```python
from build123d import *

# Parameters (mm, degrees)
BOSS_EXTRUDE1_DEPTH = 90
CUT_EXTRUDE1_DEPTH  = 385.317577012
SHELL3_T            = -10
BOSS_EXTRUDE2_START = -10
BOSS_EXTRUDE2_DEPTH = 10
SKETCH9_W           = 180
SKETCH9_H           = 60
BOSS_EXTRUDE3_DEPTH = 220
SKETCH9_4_W         = 180
SKETCH9_4_H         = 60
CUT_EXTRUDE3_DEPTH  = 200
SKETCH9_5_W         = 180
SKETCH9_5_H         = 60
BOSS_EXTRUDE5_DEPTH = 10
SKETCH10_W          = 190
SKETCH10_H          = 180
BOSS_EXTRUDE6_DEPTH = 70
SKETCH10_2_W        = 190
SKETCH10_2_H        = 180
CUT_EXTRUDE4_DEPTH  = 30
SKETCH10_3_W        = 190
SKETCH10_3_H        = 180
CUT_EXTRUDE5_DEPTH  = 50
SKETCH10_4_W        = 190
SKETCH10_4_H        = 180
CUT_EXTRUDE6_DEPTH  = 60


with BuildPart() as part:
    # Sketch1 → Boss-Extrude1 (new body)
    with BuildSketch(Plane(origin=(0, 0, 0), x_dir=(1, 0, 0), z_dir=(0, 1, 0))):
        with BuildLine():
            Line((0, 100), (0, -100))
            Line((0, -100), (200, -100))
            ThreePointArc((200, -100), (294.339811321, -72.943698113), (360, 0))
            ThreePointArc((360, 0), (294.339811321, 72.943698113), (200, 100))
            Line((200, 100), (0, 100))
        make_face()
    extrude(amount=BOSS_EXTRUDE1_DEPTH)

    # Sketch2 → Cut-Extrude1 (cut, through all)
    with BuildSketch(Plane.ZY):
        Polygon((-100, 0), (0, 0), (-100, 20), align=None)
        Polygon((0, 0), (100, 20), (100, 0), align=None)
    extrude(amount=-CUT_EXTRUDE1_DEPTH, mode=Mode.SUBTRACT)

    # Shell3
    shell3_openings = [part.faces().sort_by_distance(p)[0] for p in [
        (159.417640867, 90, 0),
    ]]
    offset(amount=SHELL3_T, openings=shell3_openings, kind=Kind.INTERSECTION)

    # Sketch6 → Boss-Extrude2 (add)
    with BuildSketch(Plane(origin=(0, 90, 0), x_dir=(1, 0, 0), z_dir=(0, 1, 0)).offset(BOSS_EXTRUDE2_START)):
        with BuildLine():
            Line((200, 90), (200, -90))
            ThreePointArc((200, -90), (286.948260477, -65.749782609), (348.795161212, 0))
            ThreePointArc((348.795161212, 0), (286.948260477, 65.749782609), (200, 90))
        make_face()
    extrude(amount=BOSS_EXTRUDE2_DEPTH)

    # Sketch9 → Boss-Extrude3 (add)
    with BuildSketch(Plane.ZY):
        with Locations((0, 50)):
            Rectangle(SKETCH9_W, SKETCH9_H)
    extrude(amount=-BOSS_EXTRUDE3_DEPTH)

    # Sketch9_4 → Cut-Extrude3 (cut)
    with BuildSketch(Plane.ZY):
        with Locations((0, 50)):
            Rectangle(SKETCH9_4_W, SKETCH9_4_H)
    extrude(amount=-CUT_EXTRUDE3_DEPTH, mode=Mode.SUBTRACT)

    # Sketch9_5 → Boss-Extrude5 (add)
    with BuildSketch(Plane.ZY):
        with Locations((0, 50)):
            Rectangle(SKETCH9_5_W, SKETCH9_5_H)
    extrude(amount=-BOSS_EXTRUDE5_DEPTH)

    # Sketch10 → Boss-Extrude6 (add)
    with BuildSketch(Plane(origin=(0, 90, 0), x_dir=(1, 0, 0), z_dir=(0, 1, 0))):
        with Locations((105, 0)):
            Rectangle(SKETCH10_W, SKETCH10_H)
    extrude(amount=-BOSS_EXTRUDE6_DEPTH)

    # Sketch10_2 → Cut-Extrude4 (cut)
    with BuildSketch(Plane(origin=(0, 90, 0), x_dir=(1, 0, 0), z_dir=(0, 1, 0))):
        with Locations((105, 0)):
            Rectangle(SKETCH10_2_W, SKETCH10_2_H)
    extrude(amount=-CUT_EXTRUDE4_DEPTH, mode=Mode.SUBTRACT)

    # Sketch10_3 → Cut-Extrude5 (cut)
    with BuildSketch(Plane(origin=(0, 90, 0), x_dir=(1, 0, 0), z_dir=(0, 1, 0))):
        with Locations((105, 0)):
            Rectangle(SKETCH10_3_W, SKETCH10_3_H)
    extrude(amount=-CUT_EXTRUDE5_DEPTH, mode=Mode.SUBTRACT)

    # Sketch10_4 → Cut-Extrude6 (cut)
    with BuildSketch(Plane(origin=(0, 90, 0), x_dir=(1, 0, 0), z_dir=(0, 1, 0))):
        with Locations((105, 0)):
            Rectangle(SKETCH10_4_W, SKETCH10_4_H)
    extrude(amount=-CUT_EXTRUDE6_DEPTH, mode=Mode.SUBTRACT)


solid = part.part
```
The model under review builds one solid part; all positions refer to its coordinate system, in mm. A direction names the side the tool comes from. Round coordinates to 2 decimals unless told otherwise and drop trailing zeros. Order: outer loops, then holes, each group sorted by start corner. A loop starts at its lowest first (then second) coordinate and runs counter-clockwise, first axis right, second up. Notation, with made-up numbers: (67.25, -39) -> (76.25, -39) arc R8 ccw to (76.25, -24) -> close; hole circle Ø8 at (33.5, 45.25). An arc over 180 degrees is marked (long way). Use a Markdown table: item, result.
Q1. We need section C-C on x = 176.5. Write out the cut boundary in (y, z), then the cut area to 3 significant figures.
Values:
| item | result |
|---|---|
| outline | (0, 0) -> (20, -100) -> (90, -100) -> (90, -90) -> (30, -90) -> (30, 90) -> (90, 90) -> (90, 100) -> (20, 100) -> close; hole (10.2, 0) -> (20, -49.01) -> (20, 49.01) -> close |
| area | 4,720 mm^2 |
Q2. Clearance check with flat-ended pins moving along their axes: P1, Ø5, axis at x = 265, z = 16.5, coming from the -Y side; P2, Ø5, axis at x = 291.5, z = 15, coming from the -Y side; P3, Ø6, axis at x = 163, z = -61, coming from the +Y side. State where each tip first meets the part, or that it passes through.
Values:
| item | result |
|---|---|
| P1 | stops at y = 2.8 |
| P2 | stops at y = 2.5 |
| P3 | stops at y = 30 |
Q3. Mouldability with a two-part tool opening along Z and no side actions: class faces 4 (the cylindrical face through (293.156, 54.37, 73.677)), 5 (the flat face through (177.48, 9.86, -49.3)), 6 (the flat face through (177, 15, 24)), 7 (the flat face through (0, 46, -1)) as +Z half, -Z half, draft (parallel to the pull), parting line (faces both ways), or undercut.
Values:
| item | result |
|---|---|
| face 4 | +Z half |
| face 5 | -Z half |
| face 6 | undercut |
| face 7 | draft |
Q4. We need section D-D on y = 14.5. Write out the cut boundary in (x, z).
Values:
| item | result |
|---|---|
| outline | (0, -72.5) -> (295.05, -72.5) arc R178 ccw to (360, 0) arc R178 ccw to (295.05, 72.5) -> (0, 72.5) -> close; hole (10, -21.51) -> (335.36, -21.51) arc R168 ccw to (348.8, 0) arc R168 ccw to (335.36, 21.51) -> (10, 21.51) -> close |
Q5. We need section A-A on y = 76.5. Write out the cut boundary in (x, z).
Values:
| item | result |
|---|---|
| outline | (0, -100) -> (200, -100) arc R178 ccw to (360, 0) arc R178 ccw to (200, 100) -> (0, 100) -> close; hole (10, -90) -> (200, -90) -> (200, 90) -> (10, 90) -> close; hole (220, -88.81) arc R168 ccw to (348.8, 0) arc R168 ccw to (220, 88.81) -> close |
Q6. For line 1 (Z direction, x = 21, y = 44); line 2 (X direction, y = 58, z = 44.5); line 3 (X direction, y = 41, z = 55), list the stretches that pass through material, from the lowest coordinate up.
Values:
| item | result |
|---|---|
| line 1 | z = -100 to -90, 90 to 100 |
| line 2 | x = 0 to 10, 200 to 220, 314.97 to 329.14 |
| line 3 | x = 0 to 10, 200 to 220, 302.64 to 318.3 |
Q7. We need section B-B on z = 73. Write out the cut boundary in (x, y).
Values:
| item | result |
|---|---|
| outline | (0, 14.6) -> (294.25, 14.6) -> (294.25, 90) -> (200, 90) -> (200, 30) -> (10, 30) -> (10, 90) -> (0, 90) -> close; hole (220, 24.8) -> (273.64, 24.8) -> (273.64, 80) -> (220, 80) -> close |
Q8. Tool access review of faces 1 (the flat face through (104, 60, -90)), 2 (the flat face through (269, 80, -1)), 3 (the cylindrical face through (295.52, 54.37, -72.2)): name each direction out of +Z, -Z, +X, -X, +Y, -Y from which nothing blocks a thin tool from reaching the whole face with its end or side.
Values:
| item | result |
|---|---|
| face 1 | +Y |
| face 2 | none |
| face 3 | -Z, +X, +Y, -Y |
